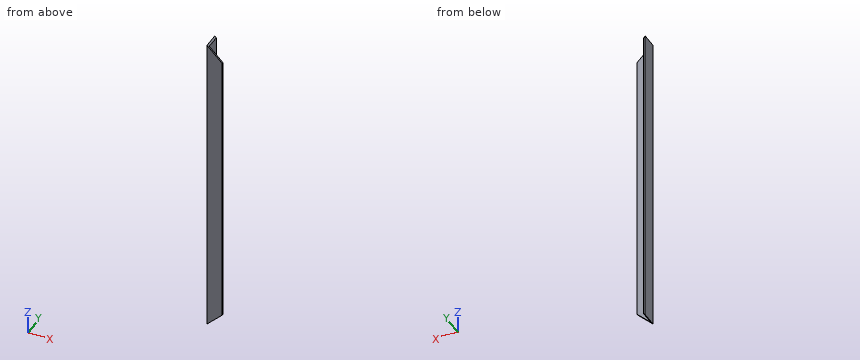
```python
from build123d import *

# Parameters (mm, degrees)
BOSS_EXTRUDE1_DEPTH = 410
CUT_EXTRUDE1_DEPTH  = 21


with BuildPart() as part:
    # Sketch1 → Boss-Extrude1 (new body)
    with BuildSketch(Plane.XY):
        Polygon((0, 20), (0, 0), (20, 0), (20, 2), (2, 2), (2, 20), align=None)
    extrude(amount=BOSS_EXTRUDE1_DEPTH)

    # Sketch2 → Cut-Extrude1 (cut, through all)
    with BuildSketch(Plane(origin=(0, 20, 0), x_dir=(1, 0, 0), z_dir=(0, 1, 0))):
        Polygon((0, 0), (20, -20), (20, 0), align=None)
        Polygon((0, -410), (20, -390), (20, -410), align=None)
    extrude(amount=-CUT_EXTRUDE1_DEPTH, mode=Mode.SUBTRACT)


solid = part.part
```
Model file for the job. Use its own axes, mm. Round coordinates to 2 decimals unless told otherwise and drop trailing zeros. Loops run counter-clockwise (first coordinate to the right, second up) from the corner with the lowest first, then second, coordinate; pieces in that order, holes last. Notation, with made-up numbers: M 56,1.5 L 94,1.5 A13 cw 94,7.5 Z; hole C 22.5,-33 d4. An arc over 180 degrees is marked long. Put each result on its own line as item: value. Start each with the question number.
Item 1: Drop flat-ended pins along their axis: P1, Ø6, axis at x = 10.5, z = 347, coming from the -Y side; P2, Ø12, axis at x = 7, y = 9, coming from the -Z side; P3, Ø10, axis at x = 12, y = 6, coming from the +Z side; P4, Ø3, axis at x = 5.5, z = 124, coming from the +Y side. Give the stop position or say it passes through.
Item 2: Drill centre line: line 1 along X through (y, z) = (9, 315.5). Where is it in solid material? Low to high.
Item 3: Cut at C-C (y = 8.25). List the corners of the cut face in (x, z).
Item 4: Cut at A-A (z = 172). List the corners of the cut face in (x, y).
Item 5: Cut at B-B (x = 8.75). List the corners of the cut face in (y, z).
Answer block:
1. P1: y = 0
1. P2: z = 1
1. P3: z = 401
1. P4: y = 2
2. line 1: 0 to 2
3. outline: M 0,0 L 2,2 L 2,408 L 0,410 Z
4. outline: M 0,0 L 20,0 L 20,2 L 2,2 L 2,20 L 0,20 Z
5. outline: M 0,8.75 L 2,8.75 L 2,401.25 L 0,401.25 Z
